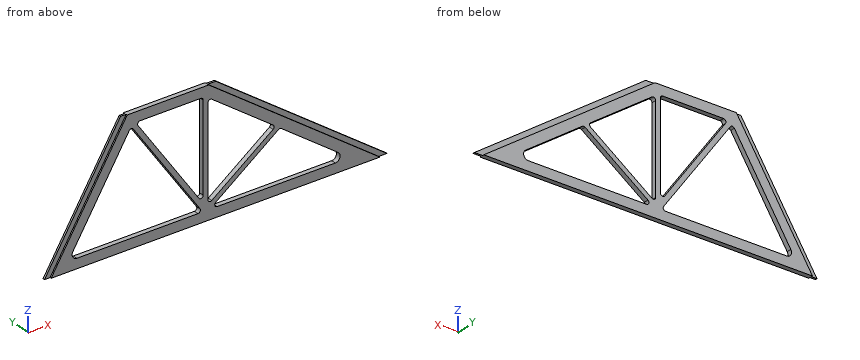
from build123d import *

# Parameters (mm, degrees)
BOSS_EXTRUDE1_DEPTH      = 3.175
BOSS_EXTRUDE1_DEPTH_BACK = 3.175
CUT_EXTRUDE1_DEPTH       = 1.905
CUT_EXTRUDE2_DEPTH       = 6.35
BOSS_EXTRUDE2_DEPTH      = 6.35
FILLET1_R                = 3.175
FILLET2_R                = 6.35


with BuildPart() as part:
    # CS path → Boss-Extrude1 (new, two sides: drawn at the far end of the back side and taken through both)
    with BuildSketch(Plane(origin=(0, 0, 0), x_dir=(1, 0, 0), z_dir=(0, 1, 0)).offset(-BOSS_EXTRUDE1_DEPTH_BACK)):
        Polygon((-228.6, 0), (228.6, 0), (0, -163.068), (-127, -163.068), align=None)
    extrude(amount=BOSS_EXTRUDE1_DEPTH + BOSS_EXTRUDE1_DEPTH_BACK)

    # Sketch1 → Cut-Extrude1 (cut)
    with BuildSketch(Plane(origin=(0, 3.175, 0), x_dir=(1, 0, 0), z_dir=(0, 1, 0))):
        Polygon((-228.6, 0), (-127, -163.068), (-119.518322882, -163.068), (-221.118322882, 0), align=None)
        Polygon((0, -163.068), (228.6, 0), (217.665386403, 0), (-10.934613597, -163.068), align=None)
    cut_extrude1 = extrude(amount=-CUT_EXTRUDE1_DEPTH, mode=Mode.SUBTRACT)

    # Mirror1: Cut-Extrude1 across plane
    add(cut_extrude1.mirror(Plane.ZX), mode=Mode.SUBTRACT)

    # Sketch2 → Cut-Extrude2 (cut)
    with BuildSketch(Plane(origin=(0, 3.175, 0), x_dir=(1, 0, 0), z_dir=(0, 1, 0))):
        Polygon((-198.24219606, -12.7), (177.99242089, -12.7), (-15.000102474, -150.368), (-112.467741232, -150.368), align=None)
    extrude(amount=-CUT_EXTRUDE2_DEPTH, mode=Mode.SUBTRACT)

    # Sketch3 → Boss-Extrude2 (add)
    with BuildSketch(Plane(origin=(0, 3.175, 0), x_dir=(1, 0, 0), z_dir=(0, 1, 0))):
        Polygon((-18.890288084, -12.7), (-114.288712294, -147.445341445), (-112.467741232, -150.368), (-108.577555622, -150.368), (-18.175102474, -22.679209355), (-18.175102474, -150.368), (-15.000102474, -150.368), (-11.825102474, -148.103166667), (-11.825102474, -18.864845516), (78.762505809, -83.484006092), (84.229812607, -79.583993908), (-9.532795675, -12.7), align=None)
    extrude(amount=-BOSS_EXTRUDE2_DEPTH)

    # Fillet1
    fillet1_edges = [part.edges().sort_by_distance(p)[0] for p in [
        (-18.175102474, 0, 150.368),
        (-18.175102474, 0, 22.679209355),
        (-108.577555622, 0, 150.368),
        (-114.288712294, 0, 147.445341445),
        (-18.890288084, 0, 12.7),
        (-9.532795675, 0, 12.7),
        (84.229812607, 0, 79.583993908),
        (78.762505809, 0, 83.484006092),
        (-11.825102474, 0, 18.864845516),
        (-11.825102474, 0, 148.103166667),
    ]]
    fillet(fillet1_edges, radius=FILLET1_R)

    # Fillet2
    fillet2_edges = [part.edges().sort_by_distance(p)[0] for p in [
        (-198.24219606, 0, 12.7),
        (177.99242089, 0, 12.7),
    ]]
    fillet(fillet2_edges, radius=FILLET2_R)


solid = part.part
The listing builds one solid part. Answer for the finished solid, in the listing's coordinates (mm). Coordinates: 2 decimals unless noted, no trailing zeros. Write each loop counter-clockwise with the first axis right and the second up, starting at its lowest first coordinate (ties: lowest second). Pieces come first, ordered by that corner, then holes. Notation, with made-up numbers: (-15, -33) -> (16, -33) arc R5 cw to (16, -26) -> close; hole circle Ø3 at (76, 12.25). An arc over 180 degrees is marked (long way). One line per question, with ' | ' between items.
1. Section B-B (z = 135.5) is taken. Determine the outline of the cut face in (x, y) (3 decimals), and give its area (3 significant figures).
Verdict:
outline: (-144.176, -1.27) -> (-136.695, -1.27) -> (-136.695, -3.175) -> (-121.731, -3.175) -> (-121.731, 3.175) -> (-136.695, 3.175) -> (-136.695, 1.27) -> (-144.176, 1.27) -> close; (-105.832, -3.175) -> (-98.051, -3.175) -> (-98.051, 3.175) -> (-105.832, 3.175) -> close; (-18.175, -3.175) -> (-11.825, -3.175) -> (-11.825, 3.175) -> (-18.175, 3.175) -> close; (5.843, -3.175) -> (27.712, -3.175) -> (27.712, -1.27) -> (38.647, -1.27) -> (38.647, 1.27) -> (27.712, 1.27) -> (27.712, 3.175) -> (5.843, 3.175) -> close | area: 370 mm^2
2. Section A-A (x = 69.5) is taken. Determine the outline of the cut face in (y, z) (3 decimals).
Verdict:
outline: (-3.175, 0) -> (3.175, 0) -> (3.175, 12.7) -> (-3.175, 12.7) -> close; (-3.175, 69.077) -> (3.175, 69.077) -> (3.175, 76.877) -> (-3.175, 76.877) -> close; (-3.175, 90.091) -> (3.175, 90.091) -> (3.175, 105.691) -> (1.27, 105.691) -> (1.27, 113.491) -> (-1.27, 113.491) -> (-1.27, 105.691) -> (-3.175, 105.691) -> close
3. Section D-D (x = -36) is taken. Determine the outline of the cut face in (y, z) (3 decimals).
Verdict:
outline: (-3.175, 0) -> (3.175, 0) -> (3.175, 12.7) -> (-3.175, 12.7) -> close; (-3.175, 36.867) -> (3.175, 36.867) -> (3.175, 47.856) -> (-3.175, 47.856) -> close; (-3.175, 150.368) -> (3.175, 150.368) -> (3.175, 163.068) -> (-3.175, 163.068) -> close
4. Given pin 1 Ø3 at (x, y) = (96.5, -0.5) entering from +Z; pin 2 Ø1.9 at (y, z) = (-0.5, 86) entering from +X, each flat-ended and moving along its own axis, determine where each tip first touches the part or whether it passes through.
Verdict:
pin 1: stops at z = 95.3 | pin 2: stops at x = 109.37
5. Straight lines are drawn through the part: line 1 (X direction, y = -2, z = 35); line 2 (Z direction, x = -92, y = 2.25); line 3 (Z direction, x = -8.5, y = 0.5). For each, find the intervals that lie inside material, in ascending order.
Verdict:
line 1: x = -199.31 to -184.35, -34.68 to -26.9, -18.18 to -11.83, 10.79 to 21.73, 146.73 to 168.6 | line 2: z = 0 to 12.7, 115.96 to 126.95, 150.37 to 163.07 | line 3: z = 0 to 21.86, 145.11 to 163.07
6. Section C-C (z = 70) is taken. Determine the outline of the cut face in (x, y) (3 decimals).
Verdict:
outline: (-184.986, -1.27) -> (-177.505, -1.27) -> (-177.505, -3.175) -> (-162.541, -3.175) -> (-162.541, 3.175) -> (-177.505, 3.175) -> (-177.505, 1.27) -> (-184.986, 1.27) -> close; (-59.458, -3.175) -> (-51.678, -3.175) -> (-51.678, 3.175) -> (-59.458, 3.175) -> close; (-18.175, -3.175) -> (-11.825, -3.175) -> (-11.825, 3.175) -> (-18.175, 3.175) -> close; (59.86, -3.175) -> (70.794, -3.175) -> (70.794, 3.175) -> (59.86, 3.175) -> close; (97.665, -3.175) -> (119.535, -3.175) -> (119.535, -1.27) -> (130.469, -1.27) -> (130.469, 1.27) -> (119.535, 1.27) -> (119.535, 3.175) -> (97.665, 3.175) -> close
